Can you work these out from the model? Positions are in its coordinate system, mm. Face numbers are marked on the shaded views. A direction names the side the tool comes from. Coordinates: 2 decimals unless noted, no trailing zeros. Order: outer loops, then holes, each group sorted by start corner. A loop starts at its lowest first (then second) coordinate and runs counter-clockwise, first axis right, second up. Notation, with made-up numbers: M 70,-19.75 L 84,-19.75 A32 ccw 84,8.25 Z; hole C 89,48.5 d2. An arc over 180 degrees is marked long. Answer as a JSON object with one key per item and string values.
from build123d import *

# Parameters (mm, degrees)
SKETCH_W        = 20
SKETCH_H        = 8.5
SKETCH_R        = 1.6
PAD_DEPTH       = 10
POCKET_DEPTH    = 3
SKETCH002_R     = 1.6
POCKET001_DEPTH = 5.501
FILLET_R        = 3


with BuildPart() as part:
    # Sketch → Pad (new body)
    with BuildSketch(Plane.XY):
        with Locations((0, 0.35)):
            Rectangle(SKETCH_W, SKETCH_H)
        Circle(SKETCH_R, mode=Mode.SUBTRACT)
    extrude(amount=PAD_DEPTH)

    # Sketch001 (on Face1 of Pad) → Pocket (cut)
    with BuildSketch(Plane(origin=(0, 4.6, 0), x_dir=(-1, 0, 0), z_dir=(0, 1, 0))):
        Polygon((-5.4, 1.997779), (-2.8, 3.498889), (-2.8, 6.501111), (-5.4, 8.002221), (-8, 6.501111), (-8, 3.498889), align=None)
        Polygon((5.4, 1.997779), (8, 3.498889), (8, 6.501111), (5.4, 8.002221), (2.8, 6.501111), (2.8, 3.498889), align=None)
    extrude(amount=-POCKET_DEPTH, mode=Mode.SUBTRACT)

    # Sketch002 (on Face20 of Pocket) → Pocket001 (cut, through all)
    with BuildSketch(Plane(origin=(0, 1.6, 0), x_dir=(-1, 0, 0), z_dir=(0, 1, 0))):
        with Locations((-5.4, 5)):
            Circle(SKETCH002_R)
        with Locations((5.4, 5)):
            Circle(SKETCH002_R)
    extrude(amount=-POCKET001_DEPTH, mode=Mode.SUBTRACT)

    # Fillet
    fillet_edges = [part.edges().sort_by_distance(p)[0] for p in [
        (10, 0.35, 0),
        (10, 0.35, 10),
        (-10, 0.35, 0),
        (-10, 0.35, 10),
    ]]
    fillet(fillet_edges, radius=FILLET_R)


solid = part.part
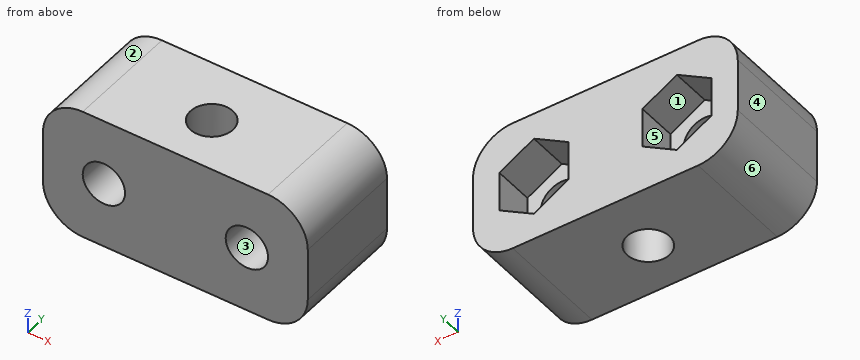
Item 1: I want a section at C-C, the plane y = -2. Write out the boundary of the cut face in (x, z), plus the area to 3 significant figures.
Answers follow:
{"outline": "M -10,3 A3 ccw -7,0 L 7,0 A3 ccw 10,3 L 10,7 A3 ccw 7,10 L -7,10 A3 ccw -10,7 Z; hole C -5.4,5 d3.2; hole C 5.4,5 d3.2", "area": "176 mm^2"}
Item 2: Please list where these lines run through material, in increasing order: line 1 (Z direction, x = -5.4, y = -1.05); line 2 (X direction, y = 0.75, z = 4.25); line 3 (X direction, y = 2.75, z = 7).
Answers follow:
{"line 1": "z = 0 to 3.4, 6.6 to 10", "line 2": "x = -10 to -6.81, -3.99 to -1.41, 1.41 to 3.99, 6.81 to 10", "line 3": "x = -10 to -7.14, -3.66 to 3.66, 7.14 to 10"}
Item 3: If we mould it in two halves opening along Z, with no side actions, what happens to the marked faces 1, 2, 3 and 4? For each: pulls with the +Z half, pulls with the -Z half, needs draft (parallel to the pull), parting line crosses it, or undercut.
Answers follow:
{"face 1": "undercut", "face 2": "pulls with the +Z half", "face 3": "undercut", "face 4": "needs draft"}
Item 4: I want a section at D-D, the plane x = -1.25. Write out the boundary of the cut face in (y, z).
Answers follow:
{"outline": "M -3.9,0 L -1,0 L -1,10 L -3.9,10 Z; M 1,0 L 4.6,0 L 4.6,10 L 1,10 Z"}
Item 5: I'm going to push a flat-ended pin straight in: pin 1 (2.5 mm diameter, centred on x = 5.4, z = 5, fed in from -Y). Where does the tip first touch, or does it pass through?
Answers follow:
{"pin 1": "passes through"}
Item 6: I want a section at B-B, the plane z = 4.25. Write out the boundary of the cut face in (x, y).
Answers follow:
{"outline": "M -10,-3.9 L -6.81,-3.9 L -6.81,1.6 L -8,1.6 L -8,4.6 L -10,4.6 Z; M -3.99,-3.9 L 3.99,-3.9 L 3.99,1.6 L 2.8,1.6 L 2.8,4.6 L -2.8,4.6 L -2.8,1.6 L -3.99,1.6 Z; M 6.81,-3.9 L 10,-3.9 L 10,4.6 L 8,4.6 L 8,1.6 L 6.81,1.6 Z; hole C 0,0 d3.2"}
Item 7: Which directions (+Z, -Z, +X, -X, +Y, -Y) give clear straight access to the entire face, cutting with the end or side of a thin tool? Please do the marked faces 5 and 6.
Answers follow:
{"face 5": "+Y", "face 6": "-Z, -X, +Y, -Y"}
Item 8: I want a section at A-A, the plane y = 0. Write out the boundary of the cut face in (x, z).
Answers follow:
{"outline": "M -10,3 A3 ccw -7,0 L -1.6,0 L -1.6,10 L -7,10 A3 ccw -10,7 Z; M 1.6,0 L 7,0 A3 ccw 10,3 L 10,7 A3 ccw 7,10 L 1.6,10 Z; hole C -5.4,5 d3.2; hole C 5.4,5 d3.2"}
